Part model, mm, in its own coordinate system. Face numbers are marked on the shaded views. Round coordinates to 2 decimals unless told otherwise and drop trailing zeros. Write each loop counter-clockwise with the first axis right and the second up, starting at its lowest first coordinate (ties: lowest second). Pieces come first, ordered by that corner, then holes. Notation, with made-up numbers: M 35.5,3.25 L 69.5,3.25 A15 cw 69.5,19.25 Z; hole C 44.5,7 d3. An arc over 180 degrees is marked long. Use one line per item in the form item = value. Start each with the question number.
Item 1: Mould opens along X. For the marked faces 1, 2 and 3 say: +X half, -X half, draft (parallel to the pull), parting line (faces both ways), or undercut.
Item 2: Cut at A-A, the plane y = 2. Give the cut face in (x, z) (3 decimals).
Item 3: Flat gauge pins, fed straight in: pin 1 Ø8 at (x, z) = (-13, -7.5) entering from -Y; pin 2 Ø3 at (x, y) = (81, 8) entering from +Z; pin 3 Ø2 at (x, z) = (69, -10) entering from +Y. Where does each tip first touch, or does it go through?
Item 4: Cut at D-D, the plane y = -17. Give the cut face in (x, z) (3 decimals), then the cut area to 3 significant figures.
Item 5: Cut at C-C, the plane z = 5.5. Give the cut face in (x, y) (3 decimals), then the cut area to 3 significant figures.
Item 6: Probe L1, parallel to X at y = 8, z = -23 (3 decimals); L2, parallel to X at y = 9, z = -2.5 (3 decimals); L3, parallel to X at y = 16.5, z = -16 (3 decimals). List the from-to ranges inside material, lowest first.
Item 7: Cut at B-B, the plane x = 83.5. Give the cut face in (y, z) (3 decimals), then the cut area to 3 significant figures.
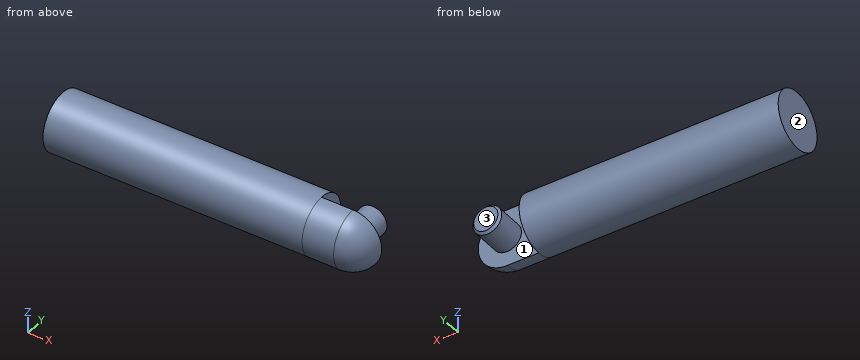
from build123d import *

# Parameters (mm, degrees)
F0_W     = 171.45
F0_H     = 19.05
F3_DEPTH = 20.828
F5_ANGLE = 90
F6_R     = 9.525
F7_DEPTH = 20.828
F8_SIZE  = 1.524


with BuildPart() as f1:
    # F0 (on Front) → F1 (revolve)
    with BuildSketch(Plane.XZ):
        Rectangle(F0_W, F0_H)
    revolve(axis=Axis((0, 0, -9.525), (1, 0, 0)))

    # F2 (on face) → F3 (join)
    with BuildSketch(Plane.YZ.offset(85.725)):
        with BuildLine():
            Line((0, -28.575), (0, 9.525))
            ThreePointArc((0, 9.525), (-19.05, -9.525), (0, -28.575))
        make_face()
    extrude(amount=F3_DEPTH)

    # F4 (on face) → F5 (revolve)
    with BuildSketch(Plane.YZ.offset(106.553)):
        with BuildLine():
            ThreePointArc((0, 9.525), (-19.05, -9.525), (0, -28.575))
            Line((0, -28.575), (0, 9.525))
        make_face()
    revolve(axis=Axis((106.553, 0, -9.525), (0, 0, 1)), revolution_arc=F5_ANGLE)

    # F6 (on face) → F7 (join)
    with BuildSketch(Plane(origin=(0, 0, 0), x_dir=(-1, 0, 0), z_dir=(0, 1, 0))):
        with Locations((-106.553, -9.525)):
            Circle(F6_R)
    extrude(amount=F7_DEPTH)

    # F8
    f8_edges = [f1.edges().sort_by_distance(p)[0] for p in [
        (116.078, 20.828, -9.525),
    ]]
    chamfer(f8_edges, length=F8_SIZE)


solid = f1.part
Model answer:
q1.face_1 = undercut
q1.face_2 = -X half
q1.face_3 = draft
q2.outline = M -85.725,-28.47 L 85.725,-28.47 L 85.725,9.42 L -85.725,9.42 Z; C 106.553,-9.525 d19.05
q3.pin_1 = -19.05
q3.pin_2 = 8.38
q3.pin_3 = 19.05
q4.outline = M -85.725,-18.122 L 106.553,-18.122 A8.597 ccw 106.553,-0.928 L -85.725,-0.928 Z
q4.area = 3,420 mm²
q5.outline = M -85.725,-11.711 L 106.553,-11.711 A11.711 ccw 118.264,0 L 85.725,0 L 85.725,11.711 L -85.725,11.711 Z
q5.area = 4,370 mm²
q6.L1 = -85.725 to 85.725
q6.L2 = -85.725 to 85.725, 100.121 to 112.985
q6.L3 = -85.725 to 85.725, 99.567 to 113.539
q7.outline = C 0,-9.525 d38.1
q7.area = 1,140 mm²
